Work out the finished part from the listing and answer in its coordinate system (mm). Coordinates: 2 decimals unless noted, no trailing zeros. Order: outer loops, then holes, each group sorted by start corner. A loop starts at its lowest first (then second) coordinate and runs counter-clockwise, first axis right, second up. Notation, with made-up numbers: M -23.5,25.5 L 22.5,25.5 A29 ccw 22.5,48.5 Z; hole C -37,18 d7. An arc over 180 degrees is marked long. Use a Markdown table: item, result.
from build123d import *

# Parameters (mm, degrees)
SFAZOWANIE1_SIZE = 0.3


with BuildPart() as part:
    # Szkic1 → Obrót1 (revolve)
    with BuildSketch(Plane.XY):
        with BuildLine():
            Line((8, 0), (20, 0))
            Line((20, 0), (20, 4.749260349))
            Line((20, 4.749260349), (19.150718002, 4.749260349))
            ThreePointArc((19.150718002, 4.749260349), (13.704182219, 2.491495571), (8, 1))
            Line((8, 1), (8, 0))
        make_face()
    revolve(axis=Axis((0, 0.249260349, 0), (0, 1, 0)))

    # Sfazowanie1
    # the kernel refuses this chamfer: 0.37665047, 0.3 mm, written as the material it takes off along each edge
    with BuildSketch(Plane(origin=(0, 0, 0), x_dir=(1, 0, 0), z_dir=(0, 0, 1))) as sfazowanie1_piece_1:
        Polygon((20 - SFAZOWANIE1_SIZE, 0), (20, SFAZOWANIE1_SIZE), (20, 0), align=None)
    revolve(axis=Axis((0, 0, 0), (0, 1, 0)), mode=Mode.SUBTRACT)
    with BuildSketch(Plane(origin=(0, 0, 0), x_dir=(1, 0, 0), z_dir=(0, 0, 1))) as sfazowanie1_piece_2:
        Polygon((8, SFAZOWANIE1_SIZE), (8 + SFAZOWANIE1_SIZE, 0), (8, 0), align=None)
    revolve(axis=Axis((0, 0, 0), (0, 1, 0)), mode=Mode.SUBTRACT)
    with BuildSketch(Plane(origin=(0, 1, 0), x_dir=(1, 0, 0), z_dir=(0, 0, 1))) as sfazowanie1_piece_3:
        with BuildLine():
            Line((8.372172674, 0.072172674), (8, -SFAZOWANIE1_SIZE))
            Line((8, -SFAZOWANIE1_SIZE), (8, 0))
            ThreePointArc((8, 0), (8.192295557, 0.036865326), (8.372172674, 0.072172674))
        make_face()
    revolve(axis=Axis((0, 1, 0), (0, 1, 0)), mode=Mode.SUBTRACT)


solid = part.part
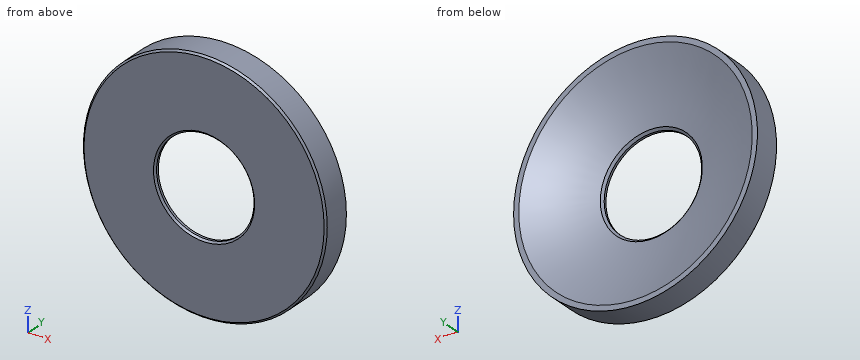
(1) Straight lines are drawn through the part: L1, parallel to Z at x = 0, y = 0.45; L2, parallel to Y at x = -10.5, z = 11. For each, find the intervals that lie inside material, in ascending order.
Conclusion:
| item | result |
|---|---|
| L1 | -20 to -8, 8 to 20 |
| L2 | 0 to 3.03 |
(2) A cutting plane is placed at A-A (x = 0). Determine the outline of the cut face in (y, z), then the cut area to 3 significant figures.
Conclusion:
| item | result |
|---|---|
| outline | M 0,-19.7 L 0.3,-20 L 4.75,-20 L 4.75,-19.15 A43 cw 1.07,-8.37 L 0.7,-8 L 0.3,-8 L 0,-8.3 Z; M 0,8.3 L 0.3,8 L 0.7,8 L 1.07,8.37 A43 cw 4.75,19.15 L 4.75,20 L 0.3,20 L 0,19.7 Z |
| area | 65.5 mm2 |
(3) Given P1, Ø1, axis at x = -4.5, z = 3.5, coming from the +Y side; P2, Ø2, axis at x = -14.5, y = 3, coming from the +Z side; P3, Ø1.5, axis at x = 6.5, z = -9, coming from the +Y side, each flat-ended and moving along its own axis, determine where each tip first touches the part or whether it passes through.
Conclusion:
| item | result |
|---|---|
| P1 | through |
| P2 | z = 14.76 |
| P3 | y = 1.91 |
(4) A cutting plane is placed at B-B (z = 0). Determine the outline of the cut face in (x, y), then the cut area to 3 significant figures.
Conclusion:
| item | result |
|---|---|
| outline | M -20,0.3 L -19.7,0 L -8.3,0 L -8,0.3 L -8,0.7 L -8.37,1.07 A43 cw -19.15,4.75 L -20,4.75 Z; M 8,0.3 L 8.3,0 L 19.7,0 L 20,0.3 L 20,4.75 L 19.15,4.75 A43 cw 8.37,1.07 L 8,0.7 Z |
| area | 65.5 mm2 |
